Geometry: see drawing. Coordinates: mm, zero at the bounding-box minimum. A direction names the side the tool comes from. Round coordinates to 2 decimals unless told otherwise and drop trailing zeros. Order: outer loops, then holes, each group sorted by start corner. A loop starts at its lowest first (then second) coordinate and runs counter-clockwise, first axis right, second up. Notation, with made-up numbers: (39.25, -8.75) -> (65.25, -8.75) arc R33 cw to (65.25, 28.25) -> close; hole circle Ø1 at (-5.5, -20.5). An arc over 180 degrees is marked (long way). Put each result on its own line as item: value.
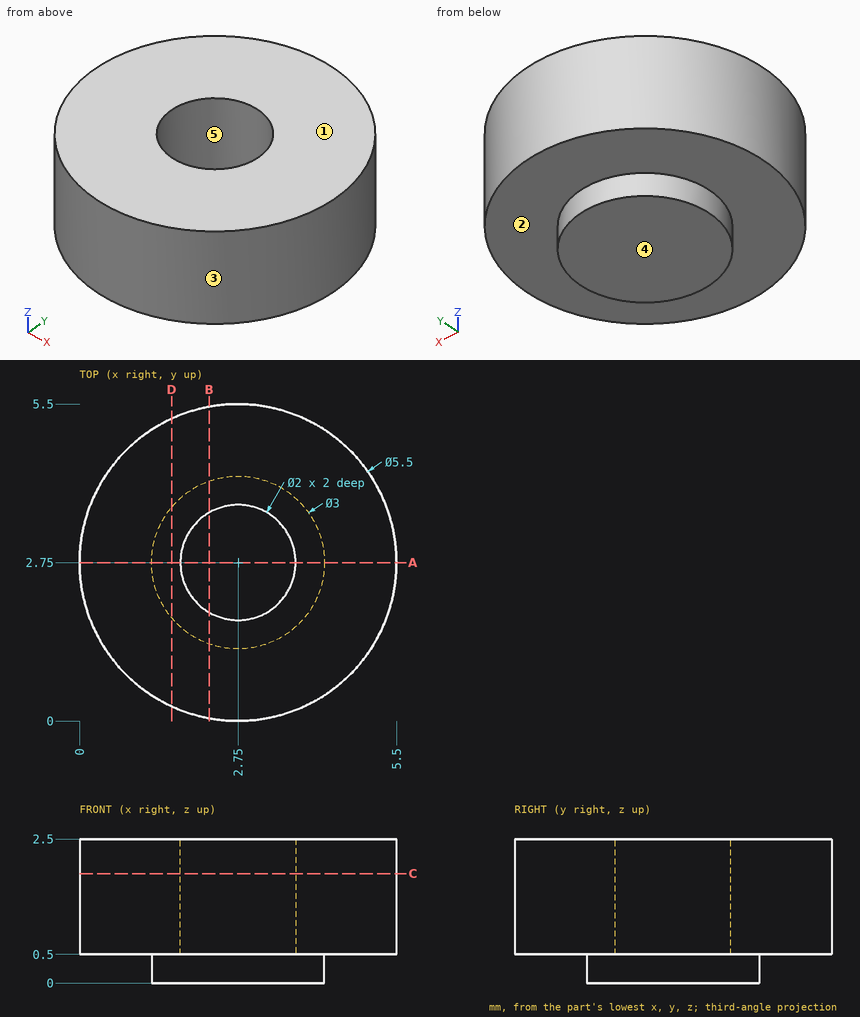
1. Cut plane B-B on x = 2.25. Return loops of the section in (y, z), and give its area (3 significant figures).
Ans:
outline: (0.05, 0.5) -> (1.34, 0.5) -> (1.34, 0) -> (4.16, 0) -> (4.16, 0.5) -> (5.45, 0.5) -> (5.45, 2.5) -> (3.62, 2.5) -> (3.62, 0.5) -> (1.88, 0.5) -> (1.88, 2.5) -> (0.05, 2.5) -> close
area: 8.77 mm²
2. Set-up query: the marked faces 1 and 2. Return all of +Z, -Z, +X, -X, +Y, -Y with unobstructed straight access to the full face (end or side cutting, diameter ignored); none if empty.
Ans:
face 1: +Z, +X, -X, +Y, -Y
face 2: -Z
3. Cut plane C-C on z = 1.9. Return loops of the section in (x, y).
Ans:
outline: circle Ø5.5 at (2.75, 2.75); hole circle Ø2 at (2.75, 2.75)
4. Contact query for flat-ended pins moving along their axis: P1, Ø1, axis at y = 4.5, z = 1.5, coming from the -X side; P2, Ø1.5, axis at y = 0.5, z = 1, coming from the +X side; P3, Ø1.6, axis at x = 2.75, y = 2.75, coming from the +Z side. Output: stop coordinate, or through.
Ans:
P1: x = 0.3
P2: x = 5.05
P3: z = 0.5
5. Material intervals for probe 1 along Y at (x, z) = (2.75, 1.3); probe 2 along Z at (x, y) = (2, 0.2); probe 3 along X at (y, z) = (3.5, 1.65), sorted ascending.
Ans:
probe 1: 0 to 1.75, 3.75 to 5.5
probe 2: 0.5 to 2.5
probe 3: 0.1 to 2.09, 3.41 to 5.4
6. Cut plane A-A on y = 2.75. Return loops of the section in (x, z).
Ans:
outline: (0, 0.5) -> (1.25, 0.5) -> (1.25, 0) -> (4.25, 0) -> (4.25, 0.5) -> (5.5, 0.5) -> (5.5, 2.5) -> (3.75, 2.5) -> (3.75, 0.5) -> (1.75, 0.5) -> (1.75, 2.5) -> (0, 2.5) -> close
7. Draft query along Y for the marked faces 3, 4 and 5. Return one class per face: +Y half, -Y half, draft (parallel to the pull), parting line (faces both ways), or undercut.
Ans:
face 3: parting line
face 4: draft
face 5: undercut
8. Cut plane D-D on x = 1.6. Return loops of the section in (y, z).
Ans:
outline: (0.25, 0.5) -> (1.79, 0.5) -> (1.79, 0) -> (3.71, 0) -> (3.71, 0.5) -> (5.25, 0.5) -> (5.25, 2.5) -> (0.25, 2.5) -> close
